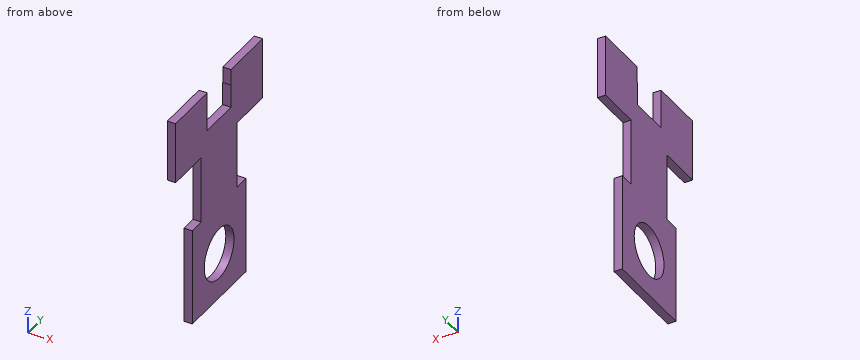
from build123d import *

# Parameters (mm, degrees)
F1_DEPTH = 4
F2_R     = 12.5
F3_DEPTH = 25


with BuildPart() as f1:
    # F0 (on Right) → F1 (new body)
    with BuildSketch(Plane.YZ):
        Polygon((-10, 53.037333), (-36.5, 53.037333), (-36.5, 23.037333), (-15, 23.037333), (-15, 0), (-15, -9.621711), (-22.5, -9.621711), (-22.5, -56.990132), (0, -56.990132), (22.5, -56.990132), (22.5, -9.621711), (15, -9.621711), (15, 0), (15, 23.037333), (36.5, 23.037333), (36.5, 53.037333), (10, 53.037333), (10, 45.139179), (9.945652, 45.139179), (9.945652, 33.913046), (-10, 33.913046), (-10, 45.139179), align=None)
    extrude(amount=F1_DEPTH)

    # F2 (on face) → F3 (cut)
    with BuildSketch(Plane.YZ.offset(4)):
        with Locations((0, -34.490132)):
            Circle(F2_R)
    extrude(amount=-F3_DEPTH, mode=Mode.SUBTRACT)


solid = f1.part
For this review, take the finished solid that the model builds, in its own axes (mm). Round coordinates to 2 decimals unless told otherwise and drop trailing zeros. Loops run counter-clockwise (first coordinate to the right, second up) from the corner with the lowest first, then second, coordinate; pieces in that order, holes last. Notation, with made-up numbers: (-14, 85.25) - (12, 85.25) arc R22 ccw to (12, 119.25) - close; hole circle Ø7 at (-29.5, -2.5). An arc over 180 degrees is marked (long way). Put each result on its own line as item: value. Start each with the question number.
1. Consider section A-A on y = 0. State the section outline as (x, z) points, plus the area to 3 significant figures.
2. For probe 1 along Y at (x, z) = (2.95, 34); probe 2 along Z at (x, y) = (1.7, -20.5); probe 3 along Z at (x, y) = (2.95, 0), list the stretches that pass through material, from the lowest coordinate up. Write a range as [from, to].
3. Consider section D-D on y = -29.5. State the section outline as (x, z) points.
4. Consider section C-C on x = 0.75. State the section outline as (y, z) points, plus the area to 3 significant figures.
5. Insertion check: P1, Ø2, axis at x = 2, y = 29, coming from the -Z side. The pin has a flat end and moves straight along its axis. Give the tip position at first contact, or say it passes through.
6. Consider section B-B on z = 38. State the section outline as (x, y) points, plus the area to 3 significant figures.
Result sheet:
1. outline: (0, -56.99) - (4, -56.99) - (4, -46.99) - (0, -46.99) - close; (0, -21.99) - (4, -21.99) - (4, 33.91) - (0, 33.91) - close
1. area: 264 mm^2
2. probe 1: [-36.5, -10], [9.95, 36.5]
2. probe 2: [-56.99, -9.62], [23.04, 53.04]
2. probe 3: [-56.99, -46.99], [-21.99, 33.91]
3. outline: (0, 23.04) - (4, 23.04) - (4, 53.04) - (0, 53.04) - close
4. outline: (-36.5, 23.04) - (-15, 23.04) - (-15, -9.62) - (-22.5, -9.62) - (-22.5, -56.99) - (22.5, -56.99) - (22.5, -9.62) - (15, -9.62) - (15, 23.04) - (36.5, 23.04) - (36.5, 53.04) - (10, 53.04) - (10, 45.14) - (9.95, 45.14) - (9.95, 33.91) - (-10, 33.91) - (-10, 53.04) - (-36.5, 53.04) - close; hole circle Ø25 at (0, -34.49)
4. area: 4,430 mm^2
5. P1: z = 23.04
6. outline: (0, -36.5) - (4, -36.5) - (4, -10) - (0, -10) - close; (0, 9.95) - (4, 9.95) - (4, 36.5) - (0, 36.5) - close
6. area: 212 mm^2
